CAD build for the part. Positions are in the model's coordinates, mm. A direction names the side the tool comes from. Give positions to 0.01 mm unless a question says otherwise; leave off trailing zeros. Loops run counter-clockwise (first coordinate to the right, second up) from the corner with the lowest first, then second, coordinate; pieces in that order, holes last. Notation, with made-up numbers: (40, 24) - (60, 24) arc R28 ccw to (60, 59) - close; hole circle Ø6 at (61, -28.75). An arc over 180 degrees is marked (long way). Return JSON: item names as keys, results as strings.
from build123d import *

# Parameters (mm, degrees)
BOSS_EXTRUDE1_DEPTH = 50
SKETCH2_R           = 5
CUT_EXTRUDE1_DEPTH  = 50
SKETCH3_R           = 3
CUT_EXTRUDE2_DEPTH  = 101


with BuildPart() as part:
    # Sketch1 → Boss-Extrude1 (new body)
    with BuildSketch(Plane.XY):
        Polygon((30, 0), (0, 0), (0, 60), (15, 60), (15, 75), (30, 75), (30, 60), (30, 50), (15, 50), (15, 20), (30, 20), align=None)
    extrude(amount=-BOSS_EXTRUDE1_DEPTH)

    # Sketch2 → Cut-Extrude1 (cut)
    with BuildSketch(Plane(origin=(30, 0, 0), x_dir=(0, 0, -1), z_dir=(1, 0, 0))):
        with Locations((25, 10)):
            Circle(SKETCH2_R)
    extrude(amount=-CUT_EXTRUDE1_DEPTH, mode=Mode.SUBTRACT)

    # Sketch3 → Cut-Extrude2 (cut)
    with BuildSketch(Plane.ZY):
        with Locations((-25, 25)):
            Circle(SKETCH3_R)
    extrude(amount=-CUT_EXTRUDE2_DEPTH, mode=Mode.SUBTRACT)


solid = part.part
1. Cut at D-D, the plane z = -17.5. Write the cut outline in (x, y), plus the area to 4 significant figures.
Values follow:
{"outline": "(0, 0) - (30, 0) - (30, 20) - (15, 20) - (15, 50) - (30, 50) - (30, 75) - (15, 75) - (15, 60) - (0, 60) - close", "area": "1,575 mm²"}
2. Cut at A-A, the plane x = 23.25. Write the cut outline in (y, z).
Values follow:
{"outline": "(0, -50) - (20, -50) - (20, 0) - (0, 0) - close; (50, -50) - (75, -50) - (75, 0) - (50, 0) - close; hole circle Ø10 at (10, -25)"}
3. Cut at C-C, the plane z = -25. Write the cut outline in (x, y), plus the area to 4 significant figures.
Values follow:
{"outline": "(0, 0) - (30, 0) - (30, 5) - (0, 5) - close; (0, 15) - (30, 15) - (30, 20) - (15, 20) - (15, 22) - (0, 22) - close; (0, 28) - (15, 28) - (15, 50) - (30, 50) - (30, 75) - (15, 75) - (15, 60) - (0, 60) - close", "area": "1,185 mm²"}
4. Drill centre lines: probe 1 along Y at (x, z) = (6.75, -25); probe 2 along Y at (x, z) = (26, -35); probe 3 along X at (y, z) = (44, -29). Where is each one in solid material? Low to high.
Values follow:
{"probe 1": "y = 0 to 5, 15 to 22, 28 to 60", "probe 2": "y = 0 to 20, 50 to 75", "probe 3": "x = 0 to 15"}
5. Drop flat-ended pins along their axis: P1, Ø7, axis at y = 25, z = -25, coming from the -X side; P2, Ø2, axis at x = 8.5, z = -44.5, coming from the +Y side; P3, Ø4, axis at y = 22.5, z = -5.5, coming from the +X side; P4, Ø5, axis at y = 66.5, z = -14, coming from the -X side. Give the stop position or say it passes through.
Values follow:
{"P1": "stops at x = 0", "P2": "stops at y = 60", "P3": "stops at x = 15", "P4": "stops at x = 15"}
6. Which spindle directions (+Z, -Z, +X, -X, +Y, -Y) get a long thin tool onto all of the face, cutting with end or side? Do faces 1 (the face through (15, 0, -25)), 2 (the face through (15, 67, -25)), 3 (the face through (15, 35, -25)). Say none if no direction does.
Values follow:
{"face 1": "+Z, -Z, +X, -X, -Y", "face 2": "+Z, -Z, -X, +Y", "face 3": "+Z, -Z, +X"}
7. Pull direction Z, two halves, no side cores. Call faces 4 (the face through (7, 25, -28)), 5 (the face through (23, 50, -25)), 6 (the face through (12, 38, 0)): +Z half, -Z half, draft (parallel to the pull), parting line (faces both ways), or undercut.
Values follow:
{"face 4": "undercut", "face 5": "draft", "face 6": "+Z half"}
8. Cut at B-B, the plane y = 10. Write the cut outline in (x, z), plus the area to 3 significant figures.
Values follow:
{"outline": "(0, -50) - (30, -50) - (30, -30) - (0, -30) - close; (0, -20) - (30, -20) - (30, 0) - (0, 0) - close", "area": "1,200 mm²"}
